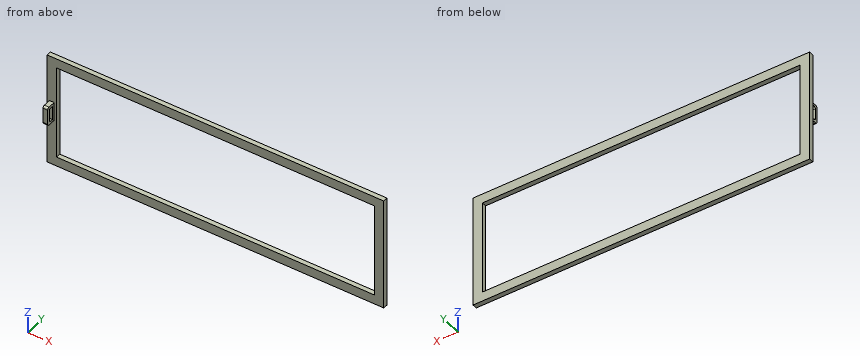
```python
from build123d import *

# Parameters (mm, degrees)
F0_W     = 914.4
F0_H     = 304.8
F0_W_2   = 863.6
F0_H_2   = 254
F1_DEPTH = 6.35
F3_DEPTH = 25.4
F5_DEPTH = 25.4
F6_R     = 5.08
F7_R     = 5.08


with BuildPart() as f1:
    # F0 (on Front) → F1 (new body, symmetric)
    with BuildSketch(Plane.XZ):
        Rectangle(F0_W, F0_H)
        Rectangle(F0_W_2, F0_H_2, mode=Mode.SUBTRACT)
    extrude(amount=F1_DEPTH, both=True)

    # F2 (on face) → F3 (join)
    with BuildSketch(Plane.XZ.offset(6.35)):
        Polygon((-438.15, 0), (-438.15, 25.4), (-450.85, 25.4), (-450.85, -25.4), (-438.15, -25.4), align=None)
    extrude(amount=F3_DEPTH)

    # F4 (on face) → F5 (cut)
    with BuildSketch(Plane(origin=(-450.85, 0, 0), x_dir=(0, -1, 0), z_dir=(-1, 0, 0))):
        Polygon((25.4, 0), (25.4, 19.05), (12.7, 19.05), (12.7, -19.05), (25.4, -19.05), align=None)
    extrude(amount=-F5_DEPTH, mode=Mode.SUBTRACT)

    # F6
    f6_edges = [f1.edges().sort_by_distance(p)[0] for p in [
        (-444.5, -25.4, 19.05),
        (-444.5, -25.4, -19.05),
    ]]
    fillet(f6_edges, radius=F6_R)

    # F7
    f7_edges = [f1.edges().sort_by_distance(p)[0] for p in [
        (-444.5, -31.75, 25.4),
        (-444.5, -31.75, -25.4),
    ]]
    fillet(f7_edges, radius=F7_R)


solid = f1.part
```
Part model, mm, in its own coordinate system. Coordinates: 2 decimals unless noted, no trailing zeros. Loops run counter-clockwise (first coordinate to the right, second up) from the corner with the lowest first, then second, coordinate; pieces in that order, holes last. Notation, with made-up numbers: (-11, 32) - (29, 32) arc R34 cw to (29, 67) - close; hole circle Ø10 at (-5, 70). An arc over 180 degrees is marked (long way). Write item = value, one per line. Start each with the question number.
Item 1: Flat gauge pins, fed straight in: pin 1 Ø12 at (y, z) = (-16, 3.5) entering from -X; pin 2 Ø4 at (x, y) = (-442.5, -17) entering from -Z; pin 3 Ø14 at (x, y) = (-447, -16) entering from +Z. Where does each tip first touch, or does it go through?
Item 2: Wall check: L1, parallel to X at y = 2, z = 19; L2, parallel to Z at x = 376.5, y = -2; L3, parallel to Y at x = 418, z = -139. Give the ranges that are in metal, low to high. Write a range as from..to.
Item 3: Cut at A-A, the plane x = 331. Give the cut face in (y, z), and give its area (3 significant figures).
Item 4: Cut at B-B, the plane z = -86.5. Give the cut face in (x, y).
The answers:
q1.pin_1 = -450.85
q1.pin_2 = -25.4
q1.pin_3 = 25.4
q2.L1 = -457.2..-431.8, 431.8..457.2
q2.L2 = -152.4..-127, 127..152.4
q2.L3 = -6.35..6.35
q3.outline = (-6.35, -152.4) - (6.35, -152.4) - (6.35, -127) - (-6.35, -127) - close; (-6.35, 127) - (6.35, 127) - (6.35, 152.4) - (-6.35, 152.4) - close
q3.area = 645 mm2
q4.outline = (-457.2, -6.35) - (-431.8, -6.35) - (-431.8, 6.35) - (-457.2, 6.35) - close; (431.8, -6.35) - (457.2, -6.35) - (457.2, 6.35) - (431.8, 6.35) - close
